from build123d import *

# Parameters (mm, degrees)
F2_R     = 7.5
F3_DEPTH = 2
F4_SIZE2 = 1.99999
F4_SIZE  = 2.99999


# Not quite as in the source:
# - a fillet or chamfer is up to 0.001 mm smaller than in the source, because OpenCascade refuses the exact size


with BuildPart() as f1:
    # F0 (on Front) → F1 (revolve)
    with BuildSketch(Plane.XZ):
        Polygon((-3.975, 0), (0, 0), (0, 7.6), (-11, 7.6), (-11, 6.6), (-3.975, 3), align=None)
    revolve(axis=Axis((0, 0, 3.8), (0, 0, 1)))

    # F2 (on face) → F3 (cut)
    with BuildSketch(Plane.XY.offset(7.6)):
        Circle(F2_R)
    extrude(amount=-F3_DEPTH, mode=Mode.SUBTRACT)

    # F4 (size 3 and 2 in the source; OpenCascade refuses exactly that, so slightly less here)
    f4_edges = [f1.edges().sort_by_distance(p)[0] for p in [
        (-7.5, 0, 5.6),
    ]]
    f4_side = f1.faces().sort_by_distance((0, 0, 5.6))[0]
    chamfer(f4_edges, length=F4_SIZE, length2=F4_SIZE2, reference=f4_side)


solid = f1.part
Source: CAD feature listing. Evaluate the final solid. Frame: model axes, mm. A direction names the side the tool comes from. Give positions to 0.01 mm unless a question says otherwise; leave off trailing zeros. Write each loop counter-clockwise with the first axis right and the second up, starting at its lowest first coordinate (ties: lowest second). Pieces come first, ordered by that corner, then holes. Notation, with made-up numbers: (77.5, 66.5) - (93.5, 66.5) arc R5 cw to (93.5, 75.5) - close; hole circle Ø1 at (84, -9.75). An arc over 180 degrees is marked (long way). Write item = value, one per line. Start each with the question number.
Q1. Pin query (flat end, axial travel): pin 1 Ø10 at (x, y) = (-1, 0) entering from +Z; pin 2 Ø12 at (x, y) = (-4, 2.5) entering from -Z; pin 3 Ø2 at (y, z) = (0.5, 4.5) entering from +X; pin 4 Ø7 at (x, y) = (0, -2) entering from +Z. Return the tip coordinate at first contact, or that it passes through.
Q2. Material intervals for probe 1 along Z at (x, y) = (-3.75, 0.75); probe 2 along X at (y, z) = (-4.25, 7); probe 3 along Y at (x, z) = (-3.5, 6), sorted ascending.
Q3. Cut plane D-D, the plane z = 3.5. Return loops of the section in (x, y), then the cut area to 3 significant figures.
Q4. Reachability of faces 1 (the flat face through (0, 0, 5.6)), 2 (the cylindrical face through (2.38, 10.74, 7.09)), 3 (the cylindrical face through (0.86, 3.88, 1.48)) from +Z, -Z, +X, -X, +Y, -Y: full face, straight path, thin tool, end or side. Return the list, or none.
Q5. Cut plane C-C, the plane z = 2. Return loops of the section in (x, y) (3 decimals).
Q6. Draft query along X for faces 4 (the conical face through (4.33, -1.795, 5.725)), 5 (the flat face through (0, 0, 0)), 6 (the conical face through (-1.992, 3.829, 3.175)). Return one class per face: +X half, -X half, draft (parallel to the pull), parting line (faces both ways), or undercut.
Computed values:
q1.pin_1 = 6.6
q1.pin_2 = 0
q1.pin_3 = 8.84
q1.pin_4 = 6.27
q2.probe_1 = 0 to 5.6
q2.probe_2 = -10.15 to -5.05, 5.05 to 10.15
q2.probe_3 = -9.18 to -3.71, 3.71 to 9.18
q3.outline = circle Ø9.9 at (0, 0)
q3.area = 77.0 mm²
q4.face_1 = +Z
q4.face_2 = +Z, -Z
q4.face_3 = -Z
q5.outline = circle Ø7.95 at (0, 0)
q6.face_4 = undercut
q6.face_5 = draft
q6.face_6 = parting line
